Solid Edge part; units mm, degrees
sketch "Sketch1" plane through (0, 0, 0) normal (0, -1, 0) x (1, 0, 0)
  line L0 (-26, -12.5) -> (26, -12.5)
  line L1 (26, -12.5) -> (26, 12.5)
  line L2 (-26, 12.5) -> (26, 12.5)
  line L3 (-26, 12.5) -> (-26, -12.5)
  dimension "D1" = 26
  dimension "D2" = 26
extrude "Protrusion1" add sketch "Sketch1" along normal blind 200
sketch "Sketch2" plane through (0, -200, 0) normal (0, -1, 0) x (1, 0, 0)
  line L0 (-16, -12.5) -> (16, -12.5)
  arc A0 (-16, -12.5) -> (16, -12.5) centre (0, -12.5) cw
  dimension "D1" = 16
extrude "Cutout1" cut sketch "Sketch2" against normal up to next
sketch "Sketch3" plane through (-26, -100, 0) normal (-1, 0, 0) x (0, -1, 0)
  circle A0 centre (55, 2.5) radius 5
  circle A1 centre (15, 2.5) radius 5
  dimension "D1" = 55
  dimension "D2" = 55
extrude "ExtrudedProtrusion_3" add sketch "Sketch3" along normal blind 19
cosmetic_thread "Thread1"
cosmetic_thread "Thread2"
hole "Hole1" at (-21, -195, -12.5) direction (0, 0, 1) diameter 6.647 end up to next
hole "Hole2" at (-21, -95, -12.5) direction (0, 0, 1) diameter 6.647 end up to next
hole "Hole3" at (21, -195, -12.5) direction (0, 0, 1) diameter 6.647 end up to next
hole "Hole4" at (21, -95, -12.5) direction (0, 0, 1) diameter 6.647 end up to next
sketch "Sketch4" plane through (-26, -100, 0) normal (-1, 0, 0) x (0, -1, 0)
  line L0 (-92, -12.5) -> (-60, -12.5)
  arc A0 (-60, -12.5) -> (-92, -12.5) centre (-76, -12.5) ccw
  dimension "D1" = 76
extrude "Cutout2" cut sketch "Sketch4" against normal up to next
sketch "Sketch5" plane through (0, 0, 0) normal (0, 1, 0) x (0, 0, -1)
  line L0 (12.5, 16) -> (12.5, 26)
  line L1 (12.5, 26) -> (-12.5, 26)
  line L2 (-12.5, 26) -> (-12.5, -26)
  line L3 (-12.5, -26) -> (12.5, -26)
  line L4 (12.5, -26) -> (12.5, -16)
  arc A0 (12.5, -16) -> (12.5, 16) centre (12.5655, 0) cw
extrude "ExtrudedProtrusion_4" add sketch "Sketch5" along normal blind 2
hole "Hole_17" at (-21, -45, -12.5) direction (0, 0, 1) diameter 6.647 end up to next
hole "Hole5" at (-21, -3, -12.5) direction (0, 0, 1) diameter 6.647 end up to next
hole "Hole_21" at (0, -173, 12.5) direction (0, 0, -1) diameter 8.376 end up to next
hole "Hole6" at (0, -78, 12.5) direction (0, 0, -1) diameter 8.376 end up to next
properties material "Stainless steel"
Part model, mm, in its own coordinate system. A direction names the side the tool comes from. Coordinates: 2 decimals unless noted, no trailing zeros. Order: outer loops, then holes, each group sorted by start corner. A loop starts at its lowest first (then second) coordinate and runs counter-clockwise, first axis right, second up. Notation, with made-up numbers: (-38.5, 88) -> (-10.5, 88) arc R28 ccw to (-10.5, 110) -> close; hole circle Ø4 at (37.25, -15). An arc over 180 degrees is marked (long way). Put each result on its own line as item: value. Start each with the question number.
(1) Pin check, flat tips, straight feed: pin 1 Ø7.5 at (x, y) = (-21, -45) entering from +Z; pin 2 Ø8 at (x, y) = (-33, -115) entering from +Z; pin 3 Ø1.5 at (y, z) = (-162.5, -8.5) entering from -X; pin 4 Ø1 at (x, y) = (-11.5, -45.5) entering from -Z. Stop position of each tip, or through.
(2) Band-saw the part on B-B (x = -21). Give the cut face in (y, z).
(3) Band-saw the part on A-A (y = -3). Give the cut face in (x, z), then the cut area to 3 significant figures.
(4) Band-saw the part on D-D (x = 21). Give the cut face in (y, z).
(5) Which spindle directions (+Z, -Z, +X, -X, +Y, -Y) get a long thin tool onto all of the face, cutting with end or side? Do faces 1 (the face through (-35.367, -150.005, 2.28)), 2 (the face through (21.15, -98.32, -0.18)). Say none if no direction does.
(6) Probe line 1 along X through (y, z) = (-195, 7.25); line 2 along Y through (x, z) = (0, 10); line 3 along Y through (x, z) = (-21, 6). List the from-to ranges inside material, lowest first. Write a range as [from, to].
(7) Mould opens along X. For faces 3 (the face through (-20, -191.83, -0.18)), 4 (the face through (0, -200, 6)), 5 (the face through (26, -100, 0)) say: pulls with the +X half, pulls with the -X half, needs draft (parallel to the pull), parting line crosses it, or undercut.
(8) Band-saw the part on C-C (y = -95). Give the cut face in (x, z), then the cut area to 3 significant figures.
Determined:
1. pin 1: stops at z = 12.5
1. pin 2: stops at z = 7.5
1. pin 3: stops at x = -26
1. pin 4: stops at z = -1.92
2. outline: (-200, -12.5) -> (-198.32, -12.5) -> (-198.32, 12.5) -> (-200, 12.5) -> close; (-191.68, -12.5) -> (-98.32, -12.5) -> (-98.32, 12.5) -> (-191.68, 12.5) -> close; (-91.68, -12.5) -> (-48.32, -12.5) -> (-48.32, 12.5) -> (-91.68, 12.5) -> close; (-41.68, -12.5) -> (-40, -12.5) arc R16 cw to (-8, -12.5) -> (-6.32, -12.5) -> (-6.32, 12.5) -> (-41.68, 12.5) -> close; (0.32, -12.5) -> (2, -12.5) -> (2, 12.5) -> (0.32, 12.5) -> close
3. outline: (-26, -12.5) -> (-24.32, -12.5) -> (-24.32, 12.5) -> (-26, 12.5) -> close; (-17.68, -12.5) -> (-16, -12.5) arc R16 cw to (16, -12.5) -> (26, -12.5) -> (26, 12.5) -> (-17.68, 12.5) -> close
3. area: 732 mm²
4. outline: (-200, -12.5) -> (-198.32, -12.5) -> (-198.32, 12.5) -> (-200, 12.5) -> close; (-191.68, -12.5) -> (-98.32, -12.5) -> (-98.32, 12.5) -> (-191.68, 12.5) -> close; (-91.68, -12.5) -> (2, -12.5) -> (2, 12.5) -> (-91.68, 12.5) -> close
5. face 1: -X
5. face 2: +Z, -Z
6. line 1: x = [-26, -24.32], [-17.68, 17.68], [24.32, 26]
6. line 2: y = [-200, -177.19], [-168.81, -82.19], [-73.81, 2]
6. line 3: y = [-200, -198.32], [-191.68, -98.32], [-91.68, -48.32], [-41.68, -6.32], [0.32, 2]
7. face 3: undercut
7. face 4: needs draft
7. face 5: pulls with the +X half
8. outline: (-26, -12.5) -> (-24.32, -12.5) -> (-24.32, 12.5) -> (-26, 12.5) -> close; (-17.68, -12.5) -> (-16, -12.5) arc R16 cw to (16, -12.5) -> (17.68, -12.5) -> (17.68, 12.5) -> (-17.68, 12.5) -> close; (24.32, -12.5) -> (26, -12.5) -> (26, 12.5) -> (24.32, 12.5) -> close
8. area: 566 mm²
